from build123d import *

# Parameters (mm, degrees)
F0_W     = 57.15
F0_H     = 101.6
F1_DEPTH = 3.175
F2_R     = 0.7874
F3_DEPTH = 3.175
F4_W     = 6.35
F4_H     = 6.35
F5_DEPTH = 3.175


with BuildPart() as f1:
    # F0 (on Top) → F1 (new body)
    with BuildSketch(Plane.XY):
        Rectangle(F0_W, F0_H)
    extrude(amount=F1_DEPTH)

    # F2 (on face) → F3 (join)
    with BuildSketch(Plane.YZ.offset(28.575)):
        with Locations((0, 1.5875)):
            Circle(F2_R)
        with Locations((25.4, 1.5875)):
            Circle(F2_R)
        with Locations((-25.4, 1.5875)):
            Circle(F2_R)
    extrude(amount=F3_DEPTH)

    # F4 (on face) → F5 (join)
    with BuildSketch(Plane(origin=(0, 0, 0), x_dir=(1, 0, 0), z_dir=(0, 0, -1))):
        with Locations((-16.764, 32.639)):
            Rectangle(F4_W, F4_H)
        with Locations((-16.764, -32.639)):
            Rectangle(F4_W, F4_H)
        with Locations((25.4, -32.639)):
            Rectangle(F4_W, F4_H)
        with Locations((25.4, 32.639)):
            Rectangle(F4_W, F4_H)
    extrude(amount=F5_DEPTH)


solid = f1.part
Model file for the job. Use its own axes, mm. A direction names the side the tool comes from. Give positions to 0.01 mm unless a question says otherwise; leave off trailing zeros. Loops run counter-clockwise (first coordinate to the right, second up) from the corner with the lowest first, then second, coordinate; pieces in that order, holes last.
Item 1: Drop flat-ended pins along their axis: P1, Ø10, axis at x = -5.5, y = -1, coming from the -Z side; P2, Ø2.5, axis at x = -16, z = -1.5, coming from the -Y side; P3, Ø3.5, axis at y = -31, z = -2, coming from the +X side (3 decimals); P4, Ø3.5, axis at x = 26, z = -1, coming from the -Y side. Give the stop position or say it passes through.
Check values:
P1: stops at z = 0
P2: stops at y = -35.81
P3: stops at x = 28.575
P4: stops at y = -50.8
Item 2: Which spindle directions (+Z, -Z, +X, -X, +Y, -Y) get a long thin tool onto all of the face, cutting with end or side? Do faces 1 (the face through (-13.589, 33, -2)), 2 (the face through (-17, -35.814, -2)), 3 (the face through (-17, 35.814, -2)), 4 (the face through (-19.939, 33, -2)), 5 (the face through (-17, -29.464, -2)). Say none if no direction does.
Check values:
face 1: -Z, +Y, -Y
face 2: -Z, +X, -X, -Y
face 3: -Z, +X, -X, +Y
face 4: -Z, -X, +Y, -Y
face 5: -Z, +X, -X
Item 3: Mould opens along Y. For faces 6 (the face through (-17, 29.464, -2)), 7 (the face through (-17, -33, -3.175)), 8 (the face through (0, -50.8, 2)) say: +Y half, -Y half, draft (parallel to the pull), parting line (faces both ways), or undercut.
Check values:
face 6: undercut
face 7: draft
face 8: -Y half
Item 4: Slice it at A-A (x = -9.5). Write the cut outline in (y, z) (3 decimals).
Check values:
outline: (-50.8, 0) - (50.8, 0) - (50.8, 3.175) - (-50.8, 3.175) - close
Item 5: Drill centre lines: line 1 along X through (y, z) = (-33.5, -0.75) (3 decimals); line 2 along Z through (x, y) = (-5.5, -23.5) (3 decimals); line 3 along X through (y, z) = (-34.5, 0.75) (3 decimals). Where is each one in solid material? Low to high.
Check values:
line 1: x = -19.939 to -13.589, 22.225 to 28.575
line 2: z = 0 to 3.175
line 3: x = -28.575 to 28.575
Item 6: Slice it at B-B (y = -11). Write the cut outline in (x, z) (3 decimals).
Check values:
outline: (-28.575, 0) - (28.575, 0) - (28.575, 3.175) - (-28.575, 3.175) - close
